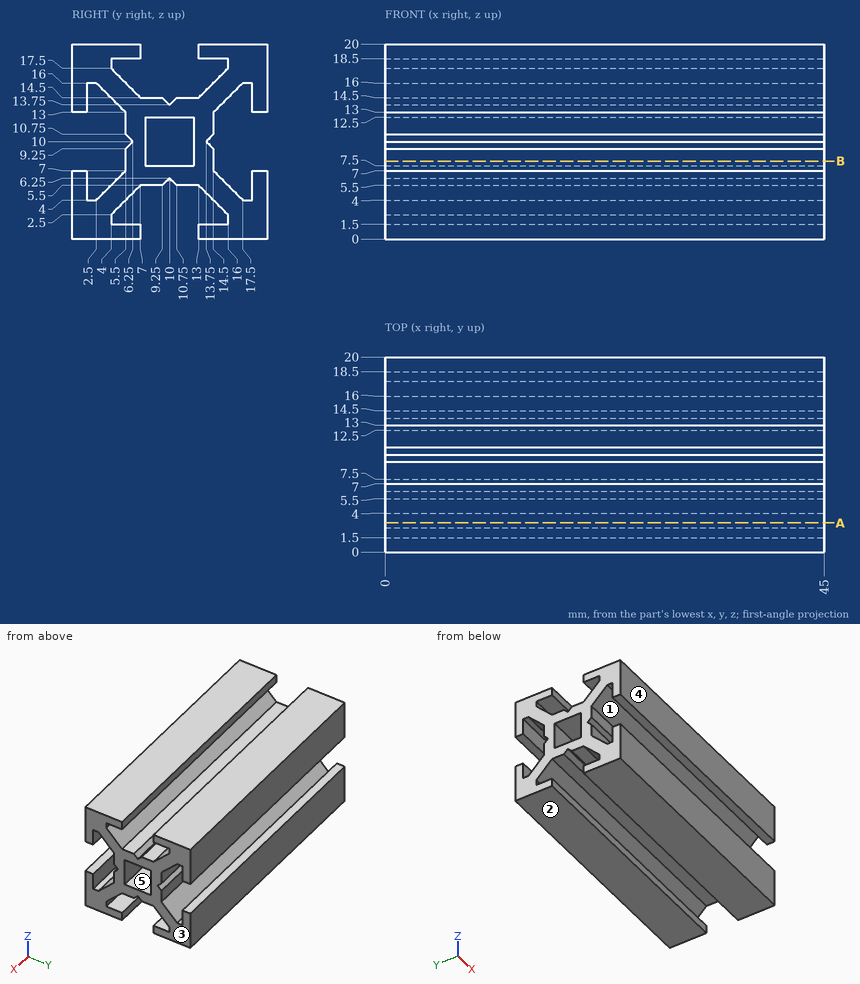
Could you check a few things on this drawing? It's one solid part, dimensions in mm from its lowest x, y, z. A direction names the side the tool comes from. Coordinates: 2 decimals unless noted, no trailing zeros. Order: outer loops, then holes, each group sorted by start corner. A loop starts at its lowest first (then second) coordinate and runs counter-clockwise, first axis right, second up. Notation, with made-up numbers: M 49.5,-25.5 L 60.5,-25.5 A36 cw 60.5,12.5 Z; hole C 64.25,48 d1. An arc over 180 degrees is marked long. Use a Markdown table: item, result. Add a question column.
Q1. I'm going to push flat-ended pins straight in: pin 1 (3.5 mm diameter, centred on x = 12.5, z = 6, fed in from -Y); pin 2 (4 mm diameter, centred on x = 22, z = 9.5, fed in from +Y); pin 3 (1.5 mm diameter, centred on x = 18.5, z = 9.5, fed in from -Y); pin 4 (1.1 mm diameter, centred on x = 33, y = 12, fed in from -Z). Where does each tip first touch, or does it pass through?
Q2. Which directions (+Z, -Z, +X, -X, +Y, -Y) give clear straight access to the entire face, cutting with the end or side of a thin tool? Please do the marked faces 4 and 5.
Q3. We'd pull the mould along Z, two halves only. Please class the marked faces 1, 2 and 3: pulls with the +Z half, pulls with the -Z half, needs draft (parallel to the pull), parting line crosses it, or undercut.
Q4. I want a section at A-A on y = 3. List the corners of the cut face in (x, z) for me.
Q5. I want a section at B-B on z = 8. List the corners of the cut face in (x, y) for me, then the cut area to 3 significant figures.
Q6. If I drill on L1, parallel to Y at x = 41, z = 11.25; L2, parallel to Z at x = 16.5, y = 4.5; L3, parallel to Y at x = 38, z = 17.75, over which ranges is the centre line in solid material (lowest first)?
Checked values:
| question | item | result |
|---|---|---|
| 1 | pin 1 | y = 0 |
| 1 | pin 2 | y = 14.5 |
| 1 | pin 3 | y = 5.5 |
| 1 | pin 4 | z = 5.5 |
| 2 | face 4 | +Z, -Z, +X, -X, -Y |
| 2 | face 5 | +X, -X |
| 3 | face 1 | undercut |
| 3 | face 2 | pulls with the -Z half |
| 3 | face 3 | needs draft |
| 4 | outline | M 0,0 L 45,0 L 45,4.5 L 0,4.5 Z; M 0,15.5 L 45,15.5 L 45,20 L 0,20 Z |
| 5 | outline | M 0,5.5 L 45,5.5 L 45,7.5 L 0,7.5 Z; M 0,12.5 L 45,12.5 L 45,14.5 L 0,14.5 Z |
| 5 | area | 180 mm² |
| 6 | L1 | 5.5 to 7.5, 12.5 to 14.5 |
| 6 | L2 | 0 to 1.5, 3 to 6, 14 to 17, 18.5 to 20 |
| 6 | L3 | 0 to 4, 16 to 20 |
